Can you work these out from the drawing? Everything is in mm from the part's minimum corner. Round coordinates to 2 decimals unless told otherwise and drop trailing zeros. Write each loop counter-clockwise with the first axis right and the second up, starting at its lowest first coordinate (ties: lowest second). Pieces come first, ordered by that corner, then holes.
Q1. I'm going to push flat-ended pins straight in: pin 1 Ø6.5 at (x, y) = (46.5, 47.35) entering from +Z; pin 2 Ø4 at (x, y) = (12.5, 59) entering from -Z; pin 3 Ø1.2 at (y, z) = (27.5, 3.5) entering from -X; pin 4 Ø0.8 at (x, z) = (58, 2.5) entering from -Y. Where does each tip first touch, or does it pass through?
Q2. If we section it at A-A (y = 47.35): Please give me the cut outline in (x, z).
Q3. If we section it at D-D (y = 28.5): Please give me the cut outline in (x, z), plus the area to 3 significant figures.
Q4. We'd pull the mould along Y, two halves only. Please class the marked faces 1 and 2: +Y half, -Y half, draft (parallel to the pull), parting line (faces both ways), or undercut.
Q5. If we section it at C-C (x = 23): Please give me the cut outline in (y, z).
Q6. If we section it at B-B (x = 46.5): Please give me the cut outline in (y, z).
Q7. Please list where these lines run through material, in increasing order: line 1 along Y through (x, z) = (46.5, 1.1); line 2 along Y through (x, z) = (71.5, 2.7); line 3 along X through (y, z) = (32, 2.9).
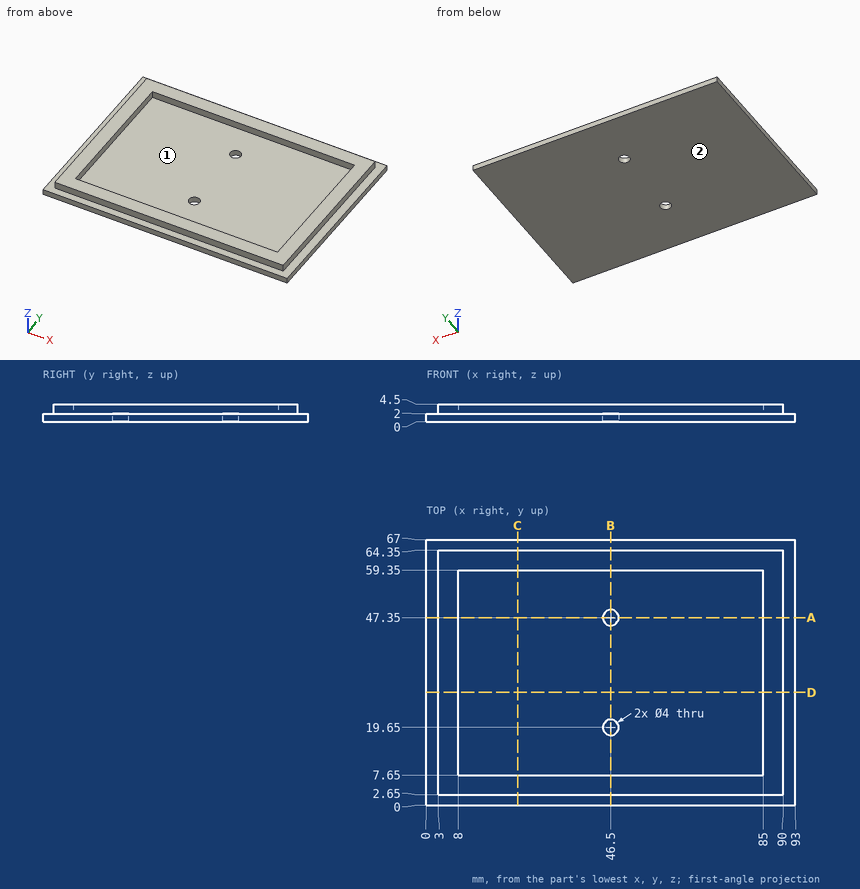
A:
1. pin 1: stops at z = 2
1. pin 2: stops at z = 0
1. pin 3: stops at x = 3
1. pin 4: stops at y = 2.65
2. outline: (0, 0) - (44.5, 0) - (44.5, 2) - (8, 2) - (8, 4.5) - (3, 4.5) - (3, 2) - (0, 2) - close; (48.5, 0) - (93, 0) - (93, 2) - (90, 2) - (90, 4.5) - (85, 4.5) - (85, 2) - (48.5, 2) - close
3. outline: (0, 0) - (93, 0) - (93, 2) - (90, 2) - (90, 4.5) - (85, 4.5) - (85, 2) - (8, 2) - (8, 4.5) - (3, 4.5) - (3, 2) - (0, 2) - close
3. area: 211 mm2
4. face 1: undercut
4. face 2: draft
5. outline: (0, 0) - (67, 0) - (67, 2) - (64.35, 2) - (64.35, 4.5) - (59.35, 4.5) - (59.35, 2) - (7.65, 2) - (7.65, 4.5) - (2.65, 4.5) - (2.65, 2) - (0, 2) - close
6. outline: (0, 0) - (17.65, 0) - (17.65, 2) - (7.65, 2) - (7.65, 4.5) - (2.65, 4.5) - (2.65, 2) - (0, 2) - close; (21.65, 0) - (45.35, 0) - (45.35, 2) - (21.65, 2) - close; (49.35, 0) - (67, 0) - (67, 2) - (64.35, 2) - (64.35, 4.5) - (59.35, 4.5) - (59.35, 2) - (49.35, 2) - close
7. line 1: y = 0 to 17.65, 21.65 to 45.35, 49.35 to 67
7. line 2: y = 2.65 to 7.65, 59.35 to 64.35
7. line 3: x = 3 to 8, 85 to 90
